For this review, use the dimensioned drawing (mm, ordinates from the lowest corner) and the shaded views. A direction names the side the tool comes from. Coordinates: 2 decimals unless noted, no trailing zeros. Order: outer loops, then holes, each group sorted by start corner. A loop starts at its lowest first (then second) coordinate and runs counter-clockwise, first axis right, second up. Notation, with made-up numbers: M 33.25,41 L 40.25,41 A17 ccw 40.25,64 Z; hole C 39.5,49.25 d1. An arc over 180 degrees is marked long. One line per item, written item: value.
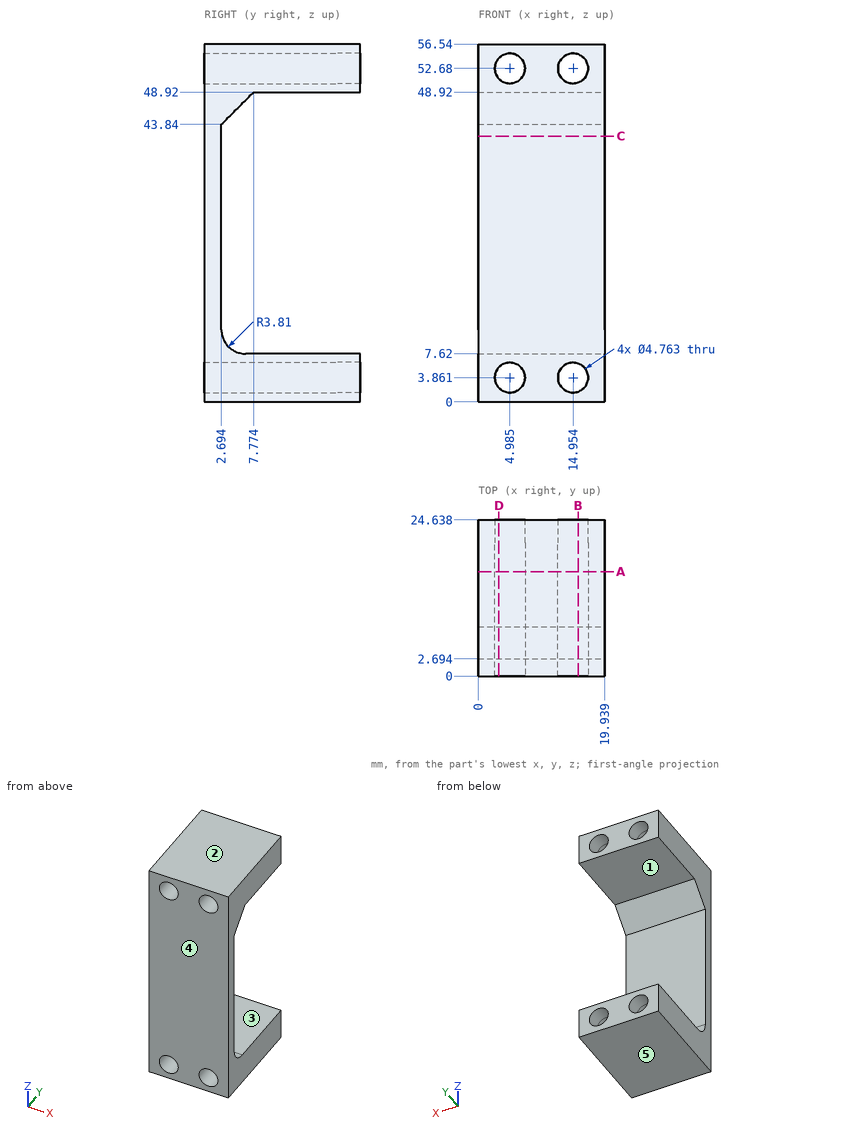
(1) Insertion check: pin 1 Ø4.5 at (x, z) = (14.95, 3.86) entering from +Y; pin 2 Ø3 at (x, z) = (15, 16.5) entering from +Y. Each pin has a flat end and moves straight along its axis. Give the tip position at first contact, or say it passes through.
Geometry results:
pin 1: passes through
pin 2: stops at y = 2.69
(2) Mouldability with a two-part tool opening along Z and no side actions: class the marked faces 3, 4 and 5 as +Z half, -Z half, draft (parallel to the pull), parting line (faces both ways), or undercut.
Geometry results:
face 3: undercut
face 4: draft
face 5: -Z half
(3) Tool access review of the marked faces 1 and 2: name each direction out of +Z, -Z, +X, -X, +Y, -Y from which nothing blocks a thin tool from reaching the whole face with its end or side.
Geometry results:
face 1: +X, -X, +Y
face 2: +Z, +X, -X, +Y, -Y
(4) We need section C-C, the plane z = 42. State the section outline as (x, y) points (1 decimal).
Geometry results:
outline: M 0,0 L 19.9,0 L 19.9,2.7 L 0,2.7 Z
(5) For L1, parallel to X at y = 4, z = 52.5; L2, parallel to Z at x = 9.25, y = 22; L3, parallel to Z at x = 14, y = 13, list the stretches that pass through material, from the lowest coordinate up.
Geometry results:
L1: x = 0 to 2.61, 7.36 to 12.58, 17.33 to 19.94
L2: z = 0 to 7.62, 48.92 to 56.54
L3: z = 0 to 1.68, 6.04 to 7.62, 48.92 to 50.5, 54.86 to 56.54
(6) We need section A-A, the plane y = 16.5. State the section outline as (x, z) points (1 decimal).
Geometry results:
outline: M 0,0 L 19.9,0 L 19.9,7.6 L 0,7.6 Z; M 0,48.9 L 19.9,48.9 L 19.9,56.5 L 0,56.5 Z; hole C 5,3.9 d4.8; hole C 5,52.7 d4.8; hole C 15,3.9 d4.8; hole C 15,52.7 d4.8
(7) We need section B-B, the plane x = 15.75. State the section outline as (y, z) points (1 decimal).
Geometry results:
outline: M 0,0 L 24.6,0 L 24.6,1.6 L 0,1.6 Z; M 0,6.1 L 24.6,6.1 L 24.6,7.6 L 6.5,7.6 A3.8 cw 2.7,11.4 L 2.7,43.8 L 7.8,48.9 L 24.6,48.9 L 24.6,50.4 L 0,50.4 Z; M 0,54.9 L 24.6,54.9 L 24.6,56.5 L 0,56.5 Z
(8) We need section D-D, the plane x = 3.25. State the section outline as (y, z) points (1 decimal), plus the area to 3 significant figures.
Geometry results:
outline: M 0,0 L 24.6,0 L 24.6,2.2 L 0,2.2 Z; M 0,5.5 L 24.6,5.5 L 24.6,7.6 L 6.5,7.6 A3.8 cw 2.7,11.4 L 2.7,43.8 L 7.8,48.9 L 24.6,48.9 L 24.6,51 L 0,51 Z; M 0,54.3 L 24.6,54.3 L 24.6,56.5 L 0,56.5 Z
area: 342 mm2
